Could you check a few things on this drawing? It's one solid part, dimensions in mm from its lowest x, y, z. Round coordinates to 2 decimals unless told otherwise and drop trailing zeros. Write each loop counter-clockwise with the first axis right and the second up, starting at its lowest first coordinate (ties: lowest second). Pieces come first, ordered by that corner, then holes. Notation, with made-up numbers: (40.5, 70) -> (65.5, 70) arc R16 ccw to (65.5, 97) -> close; hole circle Ø1 at (21, 40.25). An arc over 180 degrees is marked (long way). Return JSON: item names as keys, results as strings.
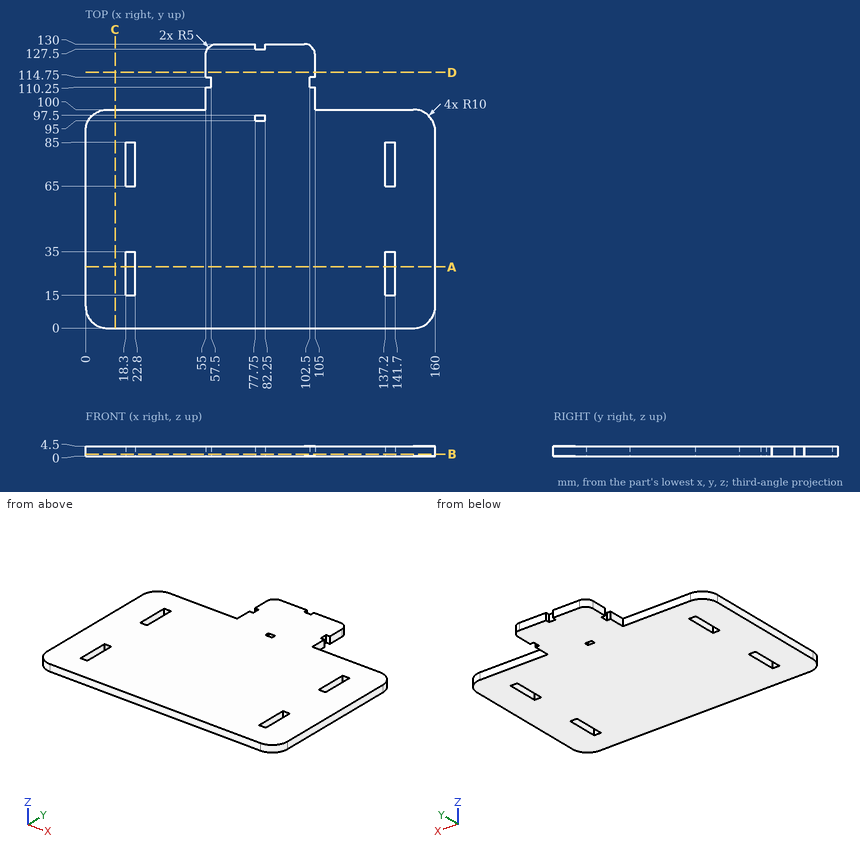
1) If I drill on probe 1 along X at (y, z) = (18.5, 2.4); probe 2 along Y at (x, z) = (22.5, 3.4); probe 3 along Y at (x, z) = (44.5, 1.85), over which ranges is the centre line in solid material (lowest first)? Write a range as [from, to].
Return value:
{"probe 1": "[0, 18.3], [22.8, 137.2], [141.7, 160]", "probe 2": "[0, 15], [35, 65], [85, 100]", "probe 3": "[0, 100]"}
2) I want a section at D-D, the plane y = 117. Please give me the cut outline in (x, z), and give its area (3 significant figures).
Return value:
{"outline": "(55, 0) -> (105, 0) -> (105, 4.5) -> (55, 4.5) -> close", "area": "225 mm²"}
3) I want a section at C-C, the plane x = 13.5. Please give me the cut outline in (y, z).
Return value:
{"outline": "(0, 0) -> (100, 0) -> (100, 4.5) -> (0, 4.5) -> close"}
4) I want a section at B-B, the plane z = 0.85. Count the separate pieces of the cut face and the enclosed holes in it, and give its area (3 significant figures).
Return value:
{"separate pieces": "1", "enclosed holes": "5", "area": "17,000 mm²"}
5) I want a section at A-A, the plane y = 28. Please give me the cut outline in (x, z).
Return value:
{"outline": "(0, 0) -> (18.3, 0) -> (18.3, 4.5) -> (0, 4.5) -> close; (22.8, 0) -> (137.2, 0) -> (137.2, 4.5) -> (22.8, 4.5) -> close; (141.7, 0) -> (160, 0) -> (160, 4.5) -> (141.7, 4.5) -> close"}
6) Will these pins go through, and if not, where does the flat tip stop? pin 1 Ø0.8 at (x, z) = (56, 1) entering from +Y; pin 2 Ø2 at (x, z) = (38, 2.5) entering from +Y; pin 3 Ø1.3 at (y, z) = (112.5, 2.5) entering from -X.
Return value:
{"pin 1": "y = 128.47", "pin 2": "y = 100", "pin 3": "x = 57.5"}
